Autodesk Inventor part; units mm, degrees
ref_plane "YZ Plane" through (0, 0, 0) normal (1, 0, 0) x (0, 1, 0)
ref_plane "XZ Plane" through (0, 0, 0) normal (0, 1, 0) x (-1, 0, 0)
ref_plane "XY Plane" through (0, 0, 0) normal (0, 0, 1) x (1, 0, 0)
sketch "Sketch1" plane through (0, 0, 0) normal (0, 1, 0) x (-1, 0, 0)
  line L0 (3.6662, 6.35) -> (7.3323, 0)
  line L1 (7.3323, 0) -> (3.6662, -6.35)
  line L2 (3.6662, -6.35) -> (-3.6662, -6.35)
  line L3 (-3.6662, -6.35) -> (-7.3323, 0)
  line L4 (-7.3323, 0) -> (-3.6662, 6.35)
  line L5 (-3.6662, 6.35) -> (3.6662, 6.35)
  point P0 (0, 0)
  point P1 (0, 0)
  dimension "d0" = 12.7
  dimension "d1" = 0
extrude "Extrusion1" add sketch "Sketch1" along normal blind 31.75
sketch "Sketch2" plane through (0, 31.75, 0) normal (0, 1, 0) x (1, 0, 0)
  circle A0 centre (0, 0) radius 9.525
  dimension "d4" = 19.05
extrude "Extrusion2" add sketch "Sketch2" along normal blind 3.175
sketch "Sketch3" plane through (0, 34.925, 0) normal (0, 1, 0) x (1, 0, 0)
  circle A0 centre (0, 0) radius 3.175
  dimension "d7" = 6.35
extrude "Extrusion3" add sketch "Sketch3" along normal blind 9.525
sketch "Sketch4" plane through (0, 44.45, 0) normal (0, 1, 0) x (1, 0, 0)
  line L0 (1.5875, -1.5875) -> (-1.5875, -1.5875)
  line L1 (-1.5875, -1.5875) -> (-1.5875, 1.5875)
  line L2 (-1.5875, 1.5875) -> (1.5875, 1.5875)
  line L3 (1.5875, 1.5875) -> (1.5875, -1.5875)
  circle A0 centre (0, 0) radius 3.175
  line L4 (1.5875, -1.5875) -> (-1.5875, 1.5875) construction
  line L5 (-1.5875, -1.5875) -> (1.5875, 1.5875) construction
  dimension "d10" = 3.175
  dimension "d11" = 3.175
extrude "Extrusion4" add sketch "Sketch4" along normal blind 19.05 contours L0 L1 L2 L3
properties part number "vex to hex adapter"
Verification items for the finished model (mm, model axes). A direction names the side the tool comes from. Round coordinates to 2 decimals unless told otherwise and drop trailing zeros. Write each loop counter-clockwise with the first axis right and the second up, starting at its lowest first coordinate (ties: lowest second). Pieces come first, ordered by that corner, then holes.
(1) Section check D-D (x = -6.5). Enter the section's corners in (y, z) (3 decimals).
Returned:
outline: (0, -1.442) - (31.75, -1.442) - (31.75, -6.962) - (34.925, -6.962) - (34.925, 6.962) - (31.75, 6.962) - (31.75, 1.442) - (0, 1.442) - close
(2) Access from +Z, -Z, +X, -X, +Y, -Y to the whole of each face (thin tool, end or side, straight path). Record for faces 5 (the flat face through (0, 54, 1.588)), 6 (the flat face through (-5.474, 15.653, 3.219)), 7 (the flat face through (0, 16, 6.35)), 8 (the flat face through (-1.588, 54, 0)).
Returned:
face 5: +Z, +X, -X, +Y
face 6: +Z, -X, -Y
face 7: +Z, +X, -X, -Y
face 8: +Z, -Z, -X, +Y
(3) Mould release check, pull along Z, two halves, no side actions. Record for faces 1 (the cylindrical face through (-0.69, 39.62, -3.1)), 2 (the flat face through (5.525, 15.653, 3.131)), 3 (the flat face through (1.588, 54, 0)), 4 (the flat face through (5.474, 15.653, -3.219)): pulls with the +Z half, pulls with the -Z half, needs draft (parallel to the pull), parting line crosses it, or undercut.
Returned:
face 1: parting line crosses it
face 2: pulls with the +Z half
face 3: needs draft
face 4: pulls with the -Z half
(4) Depth check by flat-ended pin: pin 1 Ø2.5 at (x, y) = (0, 53) entering from +Z; pin 2 Ø5.5 at (x, z) = (2.5, -4.5) entering from +Y; pin 3 Ø2.5 at (y, z) = (58.5, 0) entering from +X. Enter the tip coordinate at first touch or a pass-through.
Returned:
pin 1: stops at z = 1.59
pin 2: stops at y = 44.45
pin 3: stops at x = 1.59
(5) Section check C-C (y = 9.5). Enter the section's corners in (x, z), plus the area to 3 significant figures.
Returned:
outline: (-7.33, 0) - (-3.67, -6.35) - (3.67, -6.35) - (7.33, 0) - (3.67, 6.35) - (-3.67, 6.35) - close
area: 140 mm2
(6) Material ranges on line 1 (Y direction, x = -4.25, z = 6.5) (3 decimals); line 2 (Y direction, x = 3.25, z = -1.25) (3 decimals); line 3 (Z direction, x = 3.5, y = 20), recorded low to high.
Returned:
line 1: y = 31.75 to 34.925
line 2: y = 0 to 34.925
line 3: z = -6.35 to 6.35
(7) Section check B-B (z = -4.75). Enter the section's corners in (x, y) (3 decimals), plus the area to 3 significant figures.
Returned:
outline: (-8.256, 31.75) - (-4.59, 31.75) - (-4.59, 0) - (4.59, 0) - (4.59, 31.75) - (8.256, 31.75) - (8.256, 34.925) - (-8.256, 34.925) - close
area: 344 mm2
